Part model, mm, in its own coordinate system. A direction names the side the tool comes from. Round coordinates to 2 decimals unless told otherwise and drop trailing zeros. Order: outer loops, then holes, each group sorted by start corner. A loop starts at its lowest first (then second) coordinate and runs counter-clockwise, first axis right, second up. Notation, with made-up numbers: (-22, 34) -> (9, 34) arc R7 cw to (9, 40) -> close; hole circle Ø5 at (-27, 58.5). An arc over 180 degrees is marked (long way). Use CSV: the item, a comma, the result in double quotes.
```python
from build123d import *

# Parameters (mm, degrees)
SKETCH1_W            = 89.12
SKETCH1_H            = 85.57
BOSS_EXTRUDE1_DEPTH  = 2
SKETCH3_W            = 2
SKETCH3_H            = 30
BOSS_EXTRUDE2_DEPTH  = 85.57
SKETCH4_W            = 2
SKETCH4_H            = 30
BOSS_EXTRUDE3_DEPTH  = 85.57
SKETCH5_W            = 93.12
SKETCH5_H            = 2
BOSS_EXTRUDE4_DEPTH  = 30
SKETCH6_R            = 1.96
CUT_EXTRUDE2_DEPTH   = 30
SKETCH7_R            = 1.96
CUT_EXTRUDE3_DEPTH   = 30
SKETCH8_R            = 1.96
CUT_EXTRUDE4_DEPTH   = 30
SKETCH9_R            = 1.96
CUT_EXTRUDE5_DEPTH   = 30
SKETCH11_W           = 2
SKETCH11_H           = 12.27
BOSS_EXTRUDE5_DEPTH  = 9.4
SKETCH12_W           = 2
SKETCH12_H           = 12.27
CUT_EXTRUDE6_DEPTH   = 9.4
SKETCH13_W           = 2
SKETCH13_H           = 12.27
BOSS_EXTRUDE6_DEPTH  = 9.4
SKETCH14_W           = 2
SKETCH14_H           = 12.27
CUT_EXTRUDE7_DEPTH   = 9.4
SKETCH15_W           = 2
SKETCH15_H           = 12.27
BOSS_EXTRUDE7_DEPTH  = 9.4
SKETCH16_W           = 2
SKETCH16_H           = 12.27
CUT_EXTRUDE8_DEPTH   = 9.4
SKETCH17_W           = 2
SKETCH17_H           = 12.27
BOSS_EXTRUDE8_DEPTH  = 9.4
SKETCH18_W           = 2
SKETCH18_H           = 12.27
CUT_EXTRUDE9_DEPTH   = 9.4
BOSS_EXTRUDE9_DEPTH  = 10
SKETCH20_W           = 16
SKETCH20_H           = 42.55
BOSS_EXTRUDE10_DEPTH = 8.88
SKETCH21_W           = 16
SKETCH21_H           = 6.88
CUT_EXTRUDE10_DEPTH  = 42.55
SKETCH22_W           = 38.12
SKETCH22_H           = 9.59
BOSS_EXTRUDE11_DEPTH = 53.38
SKETCH23_W           = 34.12
SKETCH23_H           = 5.59
CUT_EXTRUDE11_DEPTH  = 53.38


with BuildPart() as part:
    # Sketch1 → Boss-Extrude1 (new body)
    with BuildSketch(Plane(origin=(0, 0, 0), x_dir=(1, 0, 0), z_dir=(0, 1, 0))):
        with Locations((44.56, 42.785)):
            Rectangle(SKETCH1_W, SKETCH1_H)
    extrude(amount=BOSS_EXTRUDE1_DEPTH)

    # Sketch3 → Boss-Extrude2 (add)
    with BuildSketch(Plane.XY):
        with Locations((-1, 15)):
            Rectangle(SKETCH3_W, SKETCH3_H)
    extrude(amount=-BOSS_EXTRUDE2_DEPTH)

    # Sketch4 → Boss-Extrude3 (add)
    with BuildSketch(Plane.XY):
        with Locations((90.12, 15)):
            Rectangle(SKETCH4_W, SKETCH4_H)
    extrude(amount=-BOSS_EXTRUDE3_DEPTH)

    # Sketch5 → Boss-Extrude4 (add)
    with BuildSketch(Plane(origin=(0, 0, 0), x_dir=(1, 0, 0), z_dir=(0, 1, 0))):
        with Locations((44.56, 86.57)):
            Rectangle(SKETCH5_W, SKETCH5_H)
    extrude(amount=BOSS_EXTRUDE4_DEPTH)

    # Sketch6 → Cut-Extrude2 (cut)
    with BuildSketch(Plane(origin=(0, 0, 0), x_dir=(1, 0, 0), z_dir=(0, 1, 0))):
        with Locations(Location((79.835, 5.755, 0), (0, 0, 90))):
            Circle(SKETCH6_R)
    extrude(amount=CUT_EXTRUDE2_DEPTH, mode=Mode.SUBTRACT)

    # Sketch7 → Cut-Extrude3 (cut)
    with BuildSketch(Plane(origin=(0, 2, 0), x_dir=(1, 0, 0), z_dir=(0, 1, 0))):
        with Locations(Location((82.285, 76.225, 0), (0, 0, 270))):
            Circle(SKETCH7_R)
    extrude(amount=-CUT_EXTRUDE3_DEPTH, mode=Mode.SUBTRACT)

    # Sketch8 → Cut-Extrude4 (cut)
    with BuildSketch(Plane(origin=(0, 0, 0), x_dir=(1, 0, 0), z_dir=(0, 1, 0))):
        with Locations(Location((6.985, 78.28, 0), (0, 0, 90))):
            Circle(SKETCH8_R)
    extrude(amount=CUT_EXTRUDE4_DEPTH, mode=Mode.SUBTRACT)

    # Sketch9 → Cut-Extrude5 (cut)
    with BuildSketch(Plane(origin=(0, 2, 0), x_dir=(1, 0, 0), z_dir=(0, 1, 0))):
        with Locations(Location((7.035, 14.85, 0), (0, 0, 270))):
            Circle(SKETCH9_R)
    extrude(amount=-CUT_EXTRUDE5_DEPTH, mode=Mode.SUBTRACT)

    # Sketch11 → Boss-Extrude5 (add)
    with BuildSketch(Plane(origin=(0, 30, 0), x_dir=(1, 0, 0), z_dir=(0, 1, 0))):
        Polygon((83.24, 12.27), (89.12, 12.27), (89.12, 14.27), (81.24, 14.27), (81.24, 12.27), align=None)
        with Locations((82.24, 6.135)):
            Rectangle(SKETCH11_W, SKETCH11_H)
    extrude(amount=-BOSS_EXTRUDE5_DEPTH)

    # Sketch12 → Cut-Extrude6 (cut)
    with BuildSketch(Plane(origin=(0, 30, 0), x_dir=(1, 0, 0), z_dir=(0, 1, 0))):
        with Locations((90.12, 6.135)):
            Rectangle(SKETCH12_W, SKETCH12_H)
    extrude(amount=-CUT_EXTRUDE6_DEPTH, mode=Mode.SUBTRACT)

    # Sketch13 → Boss-Extrude6 (add)
    with BuildSketch(Plane(origin=(0, 30, 0), x_dir=(1, 0, 0), z_dir=(0, 1, 0))):
        Polygon((83.24, 69.7), (89.12, 69.7), (89.12, 71.7), (81.24, 71.7), (81.24, 69.7), align=None)
        with Locations((82.24, 63.565)):
            Rectangle(SKETCH13_W, SKETCH13_H)
        Polygon((89.12, 55.359786784), (89.12, 57.43), (83.24, 57.43), (81.24, 57.43), (81.24, 55.359786784), align=None)
    extrude(amount=-BOSS_EXTRUDE6_DEPTH)

    # Sketch14 → Cut-Extrude7 (cut)
    with BuildSketch(Plane(origin=(0, 30, 0), x_dir=(1, 0, 0), z_dir=(0, 1, 0))):
        with Locations((90.12, 63.565)):
            Rectangle(SKETCH14_W, SKETCH14_H)
    extrude(amount=-CUT_EXTRUDE7_DEPTH, mode=Mode.SUBTRACT)

    # Sketch15 → Boss-Extrude7 (add)
    with BuildSketch(Plane(origin=(0, 30, 0), x_dir=(1, 0, 0), z_dir=(0, 1, 0))):
        Polygon((0, 71.91), (0, 69.91), (5.88, 69.91), (7.88, 69.91), (7.88, 71.91), align=None)
        with Locations((6.88, 63.775)):
            Rectangle(SKETCH15_W, SKETCH15_H)
        Polygon((5.88, 57.64), (0, 57.64), (0, 55.64), (7.88, 55.64), (7.88, 57.64), align=None)
    extrude(amount=-BOSS_EXTRUDE7_DEPTH)

    # Sketch16 → Cut-Extrude8 (cut)
    with BuildSketch(Plane(origin=(0, 30, 0), x_dir=(1, 0, 0), z_dir=(0, 1, 0))):
        with Locations((-1, 63.775)):
            Rectangle(SKETCH16_W, SKETCH16_H)
    extrude(amount=-CUT_EXTRUDE8_DEPTH, mode=Mode.SUBTRACT)

    # Sketch17 → Boss-Extrude8 (add)
    with BuildSketch(Plane(origin=(0, 30, 0), x_dir=(1, 0, 0), z_dir=(0, 1, 0))):
        Polygon((0, 14.27), (0, 12.27), (5.88, 12.27), (7.88, 12.27), (7.88, 14.27), align=None)
        with Locations((6.88, 6.135)):
            Rectangle(SKETCH17_W, SKETCH17_H)
    extrude(amount=-BOSS_EXTRUDE8_DEPTH)

    # Sketch18 → Cut-Extrude9 (cut)
    with BuildSketch(Plane(origin=(0, 30, 0), x_dir=(1, 0, 0), z_dir=(0, 1, 0))):
        with Locations((-1, 6.135)):
            Rectangle(SKETCH18_W, SKETCH18_H)
    extrude(amount=-CUT_EXTRUDE9_DEPTH, mode=Mode.SUBTRACT)

    # Sketch19 → Boss-Extrude9 (add)
    with BuildSketch(Plane(origin=(0, 30, 0), x_dir=(1, 0, 0), z_dir=(0, 1, 0))):
        Polygon((83.24, 0), (81.24, 0), (81.24, 14.27), (89.12, 14.27), (89.12, 55.359786784), (81.24, 55.359786784), (81.24, 71.7), (89.12, 71.7), (89.12, 85.57), (0, 85.57), (0, 71.91), (7.88, 71.91), (7.88, 55.64), (0, 55.64), (0, 14.27), (7.88, 14.27), (7.88, 0), (5.88, 0), (5.88, 12.27), (-2, 12.27), (-2, 57.64), (5.88, 57.64), (5.88, 69.91), (-2, 69.91), (-2, 87.57), (91.12, 87.57), (91.12, 69.7), (83.24, 69.7), (83.24, 57.43), (91.12, 57.43), (91.12, 12.27), (83.24, 12.27), align=None)
    extrude(amount=BOSS_EXTRUDE9_DEPTH)

    # Sketch20 → Boss-Extrude10 (add)
    with BuildSketch(Plane(origin=(0, 2, 0), x_dir=(1, 0, 0), z_dir=(0, 1, 0))):
        with Locations((19.1, 64.295)):
            Rectangle(SKETCH20_W, SKETCH20_H)
    extrude(amount=BOSS_EXTRUDE10_DEPTH)

    # Sketch21 → Cut-Extrude10 (cut)
    with BuildSketch(Plane.XY.offset(-43.02)):
        with Locations((19.1, 5.44)):
            Rectangle(SKETCH21_W, SKETCH21_H)
    extrude(amount=-CUT_EXTRUDE10_DEPTH, mode=Mode.SUBTRACT)

    # Sketch22 → Boss-Extrude11 (add)
    with BuildSketch(Plane.XY.offset(-85.57)):
        with Locations((30.16, 22.763941004)):
            Rectangle(SKETCH22_W, SKETCH22_H)
    extrude(amount=BOSS_EXTRUDE11_DEPTH)

    # Sketch23 → Cut-Extrude11 (cut)
    with BuildSketch(Plane.XY.offset(-32.19)):
        with Locations((30.16, 22.763941004)):
            Rectangle(SKETCH23_W, SKETCH23_H)
    extrude(amount=-CUT_EXTRUDE11_DEPTH, mode=Mode.SUBTRACT)


solid = part.part
```
(1) Which spindle directions (+Z, -Z, +X, -X, +Y, -Y) get a long thin tool onto all of the face, cutting with end or side? Do faces 4 (the face through (83.24, 30, -6)), 5 (the face through (47.22, 23, -59)), 6 (the face through (81.24, 30, -63)). Say none if no direction does.
Reply:
face 4,"+Z, +X, +Y"
face 5,"+Z"
face 6,"+Z, +Y"
(2) Probe probe 1 along Y at (x, z) = (37, -63.5); probe 2 along X at (y, z) = (21.5, -32.5); probe 3 along Y at (x, z) = (18, -55). List the from-to ranges inside material, lowest first. Write a range as [from, to].
Reply:
probe 1,"[0, 2], [17.97, 19.97], [25.56, 27.56]"
probe 2,"[-2, 0], [11.1, 13.1], [47.22, 49.22], [89.12, 91.12]"
probe 3,"[0, 2], [8.88, 10.88], [17.97, 19.97], [25.56, 27.56]"
(3) Cut at C-C, the plane z = -10.5. Give the cut face in (x, y), then the cut area to 3 significant figures.
Reply:
outline,"(-2, 0) -> (91.12, 0) -> (91.12, 20.6) -> (89.12, 20.6) -> (89.12, 2) -> (0, 2) -> (0, 20.6) -> (-2, 20.6) -> close; (5.88, 20.6) -> (7.88, 20.6) -> (7.88, 40) -> (5.88, 40) -> close; (81.24, 20.6) -> (83.24, 20.6) -> (83.24, 40) -> (81.24, 40) -> close"
area,"338 mm2"
(4) Cut at B-B, the plane x = 15.5. Give the cut face in (y, z), then the cut area to 3 significant figures.
Reply:
outline,"(0, -87.57) -> (40, -87.57) -> (40, -85.57) -> (27.56, -85.57) -> (27.56, -32.19) -> (25.56, -32.19) -> (25.56, -85.57) -> (19.97, -85.57) -> (19.97, -32.19) -> (17.97, -32.19) -> (17.97, -85.57) -> (10.88, -85.57) -> (10.88, -43.02) -> (8.88, -43.02) -> (8.88, -85.57) -> (2, -85.57) -> (2, 0) -> (0, 0) -> close"
area,"550 mm2"
(5) Drop flat-ended pins along their axis: P1, Ø1.6, axis at x = 19.5, y = 9.5, coming from the +Z side; P2, Ø3, axis at x = 6.985, z = -78.28, coming from the -Y side; P3, Ø1.5, axis at x = 15.5, y = 4.5, coming from the +Z side; P4, Ø6, axis at y = 28, z = -5.5, coming from the +X side. Give the stop position or say it passes through.
Reply:
P1,"z = -43.02"
P2,"through"
P3,"z = -85.57"
P4,"x = 83.24"
(6) Pull direction X, two halves, no side cores. Call faces 1 (the face through (44, 1, 0)), 2 (the face through (7, 20.6, -64)), 3 (the face through (91.12, 20, -44)): released by +X, released by -X, zero draft, split by the parting line, or undercut.
Reply:
face 1,"zero draft"
face 2,"undercut"
face 3,"released by +X"
(7) Cut at A-A, the plane z = -49. Give the cut face in (x, y).
Reply:
outline,"(-2, 0) -> (91.12, 0) -> (91.12, 40) -> (89.12, 40) -> (89.12, 2) -> (0, 2) -> (0, 40) -> (-2, 40) -> close; (11.1, 8.88) -> (27.1, 8.88) -> (27.1, 10.88) -> (11.1, 10.88) -> close; (11.1, 17.97) -> (49.22, 17.97) -> (49.22, 27.56) -> (11.1, 27.56) -> close; hole (13.1, 19.97) -> (47.22, 19.97) -> (47.22, 25.56) -> (13.1, 25.56) -> close"
